```python
from build123d import *

# Parameters (mm, degrees)
F0_W     = 350
F0_H     = 145
F1_DEPTH = 10
F3_D     = 6


with BuildPart() as f1:
    # F0 (on Top) → F1 (new body, symmetric)
    with BuildSketch(Plane.XY):
        Rectangle(F0_W, F0_H)
    extrude(amount=F1_DEPTH, both=True)

    # F3 (through all)
    with Locations(Plane.XZ.offset(72.5)):
        with Locations((-125, 0), (-75, 0), (75, 0), (125, 0)):
            Hole(F3_D / 2)


solid = f1.part
```
Could you check a few things on this model? Use its own coordinates, in mm. Round coordinates to 2 decimals unless told otherwise and drop trailing zeros. Write each loop counter-clockwise with the first axis right and the second up, starting at its lowest first coordinate (ties: lowest second). Pieces come first, ordered by that corner, then holes. Notation, with made-up numbers: M 83.5,89 L 116.5,89 A17 ccw 116.5,103 Z; hole C 53,42 d10. An arc over 180 degrees is marked long. Write each question's results on one line, items separated by ' | '. Start each with the question number.
1. I'm going to push a flat-ended pin straight in: pin 1 Ø3.5 at (x, z) = (125, 0) entering from +Y. Where does the tip first touch, or does it pass through?
2. Imagine slicing it at B-B on z = 0. List the corners of the cut face in (x, y) for me, and give its area (3 significant figures).
3. Thinking about a two-plate mould opening in Z: for faces 1 (the face through (-175, -1, 0)), 2 (the face through (-2, 1, 10)), 3 (the face through (-127.86, 1.02, 0.9)), which applies, +Z half, -Z half, draft (parallel to the pull), parting line (faces both ways), or undercut?
4. I need wall thicknesses on L1, parallel to X at y = 35.5, z = -0.25; L2, parallel to Z at x = -125, y = 26; L3, parallel to X at y = 26.5, z = 1. Which ranges of each line are inside material? Lowest first, please. Write a range as from..to.
5. Imagine slicing it at A-A on y = 59. List the corners of the cut face in (x, z) for me, and give its area (3 significant figures).
Result sheet:
1) pin 1: passes through
2) outline: M -175,-72.5 L -128,-72.5 L -128,72.5 L -175,72.5 Z; M -122,-72.5 L -78,-72.5 L -78,72.5 L -122,72.5 Z; M -72,-72.5 L 72,-72.5 L 72,72.5 L -72,72.5 Z; M 78,-72.5 L 122,-72.5 L 122,72.5 L 78,72.5 Z; M 128,-72.5 L 175,-72.5 L 175,72.5 L 128,72.5 Z | area: 47,300 mm^2
3) face 1: draft | face 2: +Z half | face 3: undercut
4) L1: x = -175..-127.99, -122.01..-77.99, -72.01..72.01, 77.99..122.01, 127.99..175 | L2: z = -10..-3, 3..10 | L3: x = -175..-127.83, -122.17..-77.83, -72.17..72.17, 77.83..122.17, 127.83..175
5) outline: M -175,-10 L 175,-10 L 175,10 L -175,10 Z; hole C -125,0 d6; hole C -75,0 d6; hole C 75,0 d6; hole C 125,0 d6 | area: 6,890 mm^2
